from build123d import *

# Parameters (mm, degrees)
F0_W     = 960
F0_H     = 550
F0_R     = 3
F0_R_2   = 5
F0_R_3   = 6
F0_R_4   = 7.5
F1_DEPTH = 20


with BuildPart() as f1:
    # F0 (on Top) → F1 (new body)
    with BuildSketch(Plane.XY):
        with Locations((480, -275)):
            Rectangle(F0_W, F0_H)
        with Locations((7.5, -541)):
            Circle(F0_R, mode=Mode.SUBTRACT)
        with Locations((17.5, -515)):
            Circle(F0_R, mode=Mode.SUBTRACT)
        with Locations((32, -515)):
            Circle(F0_R, mode=Mode.SUBTRACT)
        with Locations((127.5, -541)):
            Circle(F0_R_2, mode=Mode.SUBTRACT)
        with Locations((172.5, -541)):
            Circle(F0_R_2, mode=Mode.SUBTRACT)
        with Locations((127.5, -484)):
            Circle(F0_R_2, mode=Mode.SUBTRACT)
        with Locations((172.5, -484)):
            Circle(F0_R_2, mode=Mode.SUBTRACT)
        with Locations((205, -515)):
            Circle(F0_R_3, mode=Mode.SUBTRACT)
        with Locations((17.5, -455)):
            Circle(F0_R, mode=Mode.SUBTRACT)
        with Locations((265, -515)):
            Circle(F0_R_3, mode=Mode.SUBTRACT)
        with Locations((17.5, -395)):
            Circle(F0_R, mode=Mode.SUBTRACT)
        with Locations((46, -385)):
            Circle(F0_R_4, mode=Mode.SUBTRACT)
        with Locations((17.5, -335)):
            Circle(F0_R, mode=Mode.SUBTRACT)
        with Locations((787.5, -541)):
            Circle(F0_R_2, mode=Mode.SUBTRACT)
        with Locations((832.5, -541)):
            Circle(F0_R_2, mode=Mode.SUBTRACT)
        with Locations((787.5, -484)):
            Circle(F0_R_2, mode=Mode.SUBTRACT)
        with Locations((832.5, -484)):
            Circle(F0_R_2, mode=Mode.SUBTRACT)
        with Locations((952.5, -541)):
            Circle(F0_R, mode=Mode.SUBTRACT)
        with Locations((928, -515)):
            Circle(F0_R, mode=Mode.SUBTRACT)
        with Locations((942.5, -515)):
            Circle(F0_R, mode=Mode.SUBTRACT)
        with Locations((942.5, -455)):
            Circle(F0_R, mode=Mode.SUBTRACT)
        with Locations((914, -385)):
            Circle(F0_R_4, mode=Mode.SUBTRACT)
        with Locations((942.5, -395)):
            Circle(F0_R, mode=Mode.SUBTRACT)
        with Locations((942.5, -335)):
            Circle(F0_R, mode=Mode.SUBTRACT)
        with Locations((17.5, -275)):
            Circle(F0_R, mode=Mode.SUBTRACT)
        with Locations((17.5, -215)):
            Circle(F0_R, mode=Mode.SUBTRACT)
        with Locations((17.5, -155)):
            Circle(F0_R, mode=Mode.SUBTRACT)
        with Locations((46, -165)):
            Circle(F0_R_4, mode=Mode.SUBTRACT)
        with BuildLine():
            ThreePointArc((120, -175), (134.644661, -139.644661), (170, -125))
            Line((170, -125), (370, -125))
            ThreePointArc((370, -125), (405.355339, -139.644661), (420, -175))
            Line((420, -175), (420, -375))
            ThreePointArc((420, -375), (405.355339, -410.355339), (370, -425))
            Line((370, -425), (170, -425))
            ThreePointArc((170, -425), (134.644661, -410.355339), (120, -375))
            Line((120, -375), (120, -175))
        make_face(mode=Mode.SUBTRACT)
        with Locations((17.5, -95)):
            Circle(F0_R, mode=Mode.SUBTRACT)
        with Locations((17.5, -35)):
            Circle(F0_R, mode=Mode.SUBTRACT)
        with Locations((32, -35)):
            Circle(F0_R, mode=Mode.SUBTRACT)
        with Locations((7.5, -9)):
            Circle(F0_R, mode=Mode.SUBTRACT)
        with Locations((127.5, -66)):
            Circle(F0_R_2, mode=Mode.SUBTRACT)
        with Locations((172.5, -66)):
            Circle(F0_R_2, mode=Mode.SUBTRACT)
        with Locations((205, -35)):
            Circle(F0_R_3, mode=Mode.SUBTRACT)
        with Locations((127.5, -9)):
            Circle(F0_R_2, mode=Mode.SUBTRACT)
        with Locations((172.5, -9)):
            Circle(F0_R_2, mode=Mode.SUBTRACT)
        with Locations((265, -35)):
            Circle(F0_R_3, mode=Mode.SUBTRACT)
        with BuildLine():
            ThreePointArc((840, -375), (825.355339, -410.355339), (790, -425))
            Line((790, -425), (590, -425))
            ThreePointArc((590, -425), (554.644661, -410.355339), (540, -375))
            Line((540, -375), (540, -175))
            ThreePointArc((540, -175), (554.644661, -139.644661), (590, -125))
            Line((590, -125), (790, -125))
            ThreePointArc((790, -125), (825.355339, -139.644661), (840, -175))
            Line((840, -175), (840, -375))
        make_face(mode=Mode.SUBTRACT)
        with Locations((942.5, -275)):
            Circle(F0_R, mode=Mode.SUBTRACT)
        with Locations((942.5, -215)):
            Circle(F0_R, mode=Mode.SUBTRACT)
        with Locations((914, -165)):
            Circle(F0_R_4, mode=Mode.SUBTRACT)
        with Locations((942.5, -155)):
            Circle(F0_R, mode=Mode.SUBTRACT)
        with Locations((942.5, -95)):
            Circle(F0_R, mode=Mode.SUBTRACT)
        with Locations((787.5, -66)):
            Circle(F0_R_2, mode=Mode.SUBTRACT)
        with Locations((832.5, -66)):
            Circle(F0_R_2, mode=Mode.SUBTRACT)
        with Locations((787.5, -9)):
            Circle(F0_R_2, mode=Mode.SUBTRACT)
        with Locations((832.5, -9)):
            Circle(F0_R_2, mode=Mode.SUBTRACT)
        with Locations((928, -35)):
            Circle(F0_R, mode=Mode.SUBTRACT)
        with Locations((942.5, -35)):
            Circle(F0_R, mode=Mode.SUBTRACT)
        with Locations((952.5, -9)):
            Circle(F0_R, mode=Mode.SUBTRACT)
    extrude(amount=F1_DEPTH)


solid = f1.part
Geometry: final body of the model. Coordinates: model frame, mm. A direction names the side the tool comes from. Coordinates: 2 decimals unless noted, no trailing zeros. Loops run counter-clockwise (first coordinate to the right, second up) from the corner with the lowest first, then second, coordinate; pieces in that order, holes last. Notation, with made-up numbers: (14.25, 12.5) - (22.25, 12.5) arc R9 cw to (22.25, 23.5) - close; hole circle Ø1 at (87.5, 58.5). An arc over 180 degrees is marked (long way). One line per question, with ' | ' between items. Start each with the question number.
(1) Ray query, L1, parallel to X at y = -329.5, z = 15.75; L2, parallel to X at y = -65.5, z = 14; L3, parallel to Y at x = 914, z = 13.5. Return the intervals inside material, ascending. Write a range as from..to.
(2) Cut plane C-C on z = 11.5. Count the separate pieces of the cut face and the enclosed holes in it, and give its area (3 significant figures).
(3) Reachability of faces 4 (the flat face through (271, -425, 10)), 5 (the flat face through (473, -271, 20)) from +Z, -Z, +X, -X, +Y, -Y: full face, straight path, thin tool, end or side. Return the list, or none.
(4) Draft query along X for faces 1 (the cylindrical face through (404.964, -139.258, 9.86)), 2 (the flat face through (960, -279, 10)), 3 (the flat face through (0, -279, 10)). Return one class per face: +X half, -X half, draft (parallel to the pull), parting line (faces both ways), or undercut.
(5) Cut plane A-A on y = -256. Output: boundary loops of the cut face in (x, z).
(6) Cut plane B-B on x = 753. Output: boundary loops of the cut face in (y, z).
(7) First-contact query: pin 1 (5.5 mm diameter, centred on x = 17.5, y = -275, fed in from -Z). Flat tip, straight axial feed; report the tip coordinate or a pass-through.
Here are the results:
1) L1: 0..120, 420..540, 840..960 | L2: 0..122.53, 132.47..167.53, 177.47..782.53, 792.47..827.53, 837.47..960 | L3: -550..-392.5, -377.5..-172.5, -157.5..0
2) separate pieces: 1 | enclosed holes: 52 | area: 349,000 mm²
3) face 4: +Z, -Z | face 5: +Z, +X, -X, +Y, -Y
4) face 1: undercut | face 2: +X half | face 3: -X half
5) outline: (0, 0) - (120, 0) - (120, 20) - (0, 20) - close; (420, 0) - (540, 0) - (540, 20) - (420, 20) - close; (840, 0) - (960, 0) - (960, 20) - (840, 20) - close
6) outline: (-550, 0) - (-425, 0) - (-425, 20) - (-550, 20) - close; (-125, 0) - (0, 0) - (0, 20) - (-125, 20) - close
7) pin 1: through
